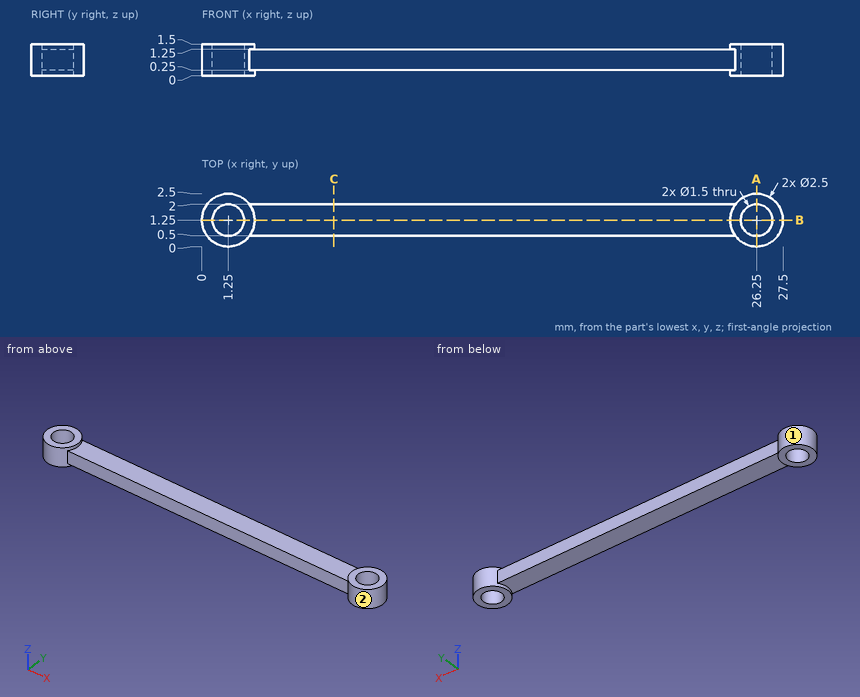
The figure shows three views and two pictorial views of one solid part (mm, origin at its lowest corner). Answer the questions. Coordinates: 2 decimals unless noted, no trailing zeros. Write each loop counter-clockwise with the first axis right and the second up, starting at its lowest first coordinate (ties: lowest second). Pieces come first, ordered by that corner, then holes. Notation, with made-up numbers: (-4.75, -28) -> (32.25, -28) arc R21 cw to (32.25, 2) -> close; hole circle Ø4 at (89.25, 4.5). An arc over 180 degrees is marked (long way). Answer as a JSON object with one key per item and string values.
Q1. Determine the mould class of the marked faces 1 and 2 for opening direction X: pulls with the +X half, pulls with the -X half, needs draft (parallel to the pull), parting line crosses it, or undercut.
The answers:
{"face 1": "undercut", "face 2": "undercut"}
Q2. The part is cut by section B-B on y = 1.25. Give the vertices of the cut face in (x, z), then the cut area to 3 significant figures.
The answers:
{"outline": "(0, 0) -> (0.5, 0) -> (0.5, 1.5) -> (0, 1.5) -> close; (2, 0) -> (2.5, 0) -> (2.5, 0.25) -> (25, 0.25) -> (25, 0) -> (25.5, 0) -> (25.5, 1.5) -> (25, 1.5) -> (25, 1.25) -> (2.5, 1.25) -> (2.5, 1.5) -> (2, 1.5) -> close; (27, 0) -> (27.5, 0) -> (27.5, 1.5) -> (27, 1.5) -> close", "area": "25.5 mm2"}
Q3. The part is cut by section C-C on x = 6.25. Give the vertices of the cut face in (y, z).
The answers:
{"outline": "(0.5, 0.25) -> (2, 0.25) -> (2, 1.25) -> (0.5, 1.25) -> close"}
Q4. Flat-ended cylindrical pins translate along their axes: pin 1 Ø0.8 at (x, y) = (17, 1.5) entering from -Z; pin 2 Ø1.2 at (x, y) = (18, 1) entering from +Z. Find the tip coordinate at first contact, or state that the pin passes through.
The answers:
{"pin 1": "stops at z = 0.25", "pin 2": "stops at z = 1.25"}
Q5. The part is cut by section A-A on x = 26.25. Give the vertices of the cut face in (y, z).
The answers:
{"outline": "(0, 0) -> (0.5, 0) -> (0.5, 1.5) -> (0, 1.5) -> close; (2, 0) -> (2.5, 0) -> (2.5, 1.5) -> (2, 1.5) -> close"}
Q6. Consider line 1 (X direction, y = 1.25, z = 0.7); line 2 (Y direction, x = 1.25, z = 1.1); line 3 (X direction, y = 1.6, z = 1.1). Determine where each line is inside the solid, lowest interval first. Write a range as [from, to].
The answers:
{"line 1": "x = [0, 0.5], [2, 25.5], [27, 27.5]", "line 2": "y = [0, 0.5], [2, 2.5]", "line 3": "x = [0.05, 0.59], [1.91, 25.59], [26.91, 27.45]"}
